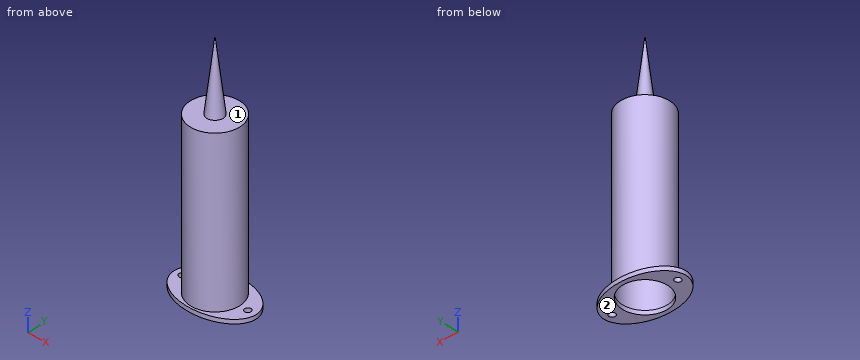
from build123d import *

# Parameters (mm, degrees)
SKETCH1_R           = 19.05
SKETCH1_R_2         = 17.4625
BOSS_EXTRUDE1_DEPTH = 123.825
SKETCH2_RX          = 31.75
SKETCH2_RY          = 20.6375
SKETCH2_R           = 17.4625
SKETCH2_R_2         = 2.413
BOSS_EXTRUDE2_DEPTH = 3.175
SKETCH3_R           = 17.4625
BOSS_EXTRUDE3_DEPTH = 4.953


with BuildPart() as part:
    # Sketch1 → Boss-Extrude1 (new body)
    with BuildSketch(Plane.XY):
        Circle(SKETCH1_R)
        Circle(SKETCH1_R_2, mode=Mode.SUBTRACT)
    extrude(amount=BOSS_EXTRUDE1_DEPTH)

    # Sketch2 → Boss-Extrude2 (add)
    with BuildSketch(Plane(origin=(0, 0, 0), x_dir=(-1, 0, 0), z_dir=(0, 0, -1))):
        with Locations((0, 0)):
            Ellipse(SKETCH2_RX, SKETCH2_RY)
        Circle(SKETCH2_R, mode=Mode.SUBTRACT)
        with Locations((25.4, 0)):
            Circle(SKETCH2_R_2, mode=Mode.SUBTRACT)
        with Locations((-25.4, 0)):
            Circle(SKETCH2_R_2, mode=Mode.SUBTRACT)
    extrude(amount=BOSS_EXTRUDE2_DEPTH)

    # Sketch3 → Boss-Extrude3 (add)
    with BuildSketch(Plane.XY.offset(123.825)):
        Circle(SKETCH3_R)
    extrude(amount=-BOSS_EXTRUDE3_DEPTH)

    # Sketch4 → Revolve1 (revolve)
    with BuildSketch(Plane(origin=(0, 0, 0), x_dir=(1, 0, 0), z_dir=(0, 1, 0))):
        Polygon((0, -123.825), (0, -177.8), (6.35, -123.825), align=None)
    revolve(axis=Axis((0, 0, 123.825), (0, 0, 1)))


solid = part.part
Model file for the job. Use its own axes, mm. Face numbers are marked on the shaded views. A direction names the side the tool comes from. Round coordinates to 2 decimals unless told otherwise and drop trailing zeros. Order: outer loops, then holes, each group sorted by start corner. A loop starts at its lowest first (then second) coordinate and runs counter-clockwise, first axis right, second up. Notation, with made-up numbers: M -38,40 L -25,40 A35 cw -25,74 Z; hole C 87.25,59 d2. An arc over 180 degrees is marked long. Write each question's results on one line, items separated by ' | '. Start each with the question number.
(1) Saw through at B-B, the plane z = 159.5. Give the cut face in (x, y).
(2) Probe probe 1 along Y at (x, z) = (0, 65.5); probe 2 along Z at (x, y) = (-3, -16.5) (3 decimals); probe 3 along Z at (x, y) = (-19, -12) (3 decimals). List the from-to ranges inside material, lowest first. Write a range as from..to.
(3) Drop flat-ended pins along their axis: pin 1 (10.5 mm diameter, centred on x = -5, y = 4.5, fed in from -Z); pin 2 (5 mm diameter, centred on y = -10.5, z = 79.5, fed in from -X); pin 3 (4.5 mm diameter, centred on x = -25.4, y = 0, fed in from +Z); pin 4 (1 mm diameter, centred on y = -6, z = 31.5, fed in from -X). Give the stop position or say it passes through.
(4) Which spindle directions (+Z, -Z, +X, -X, +Y, -Y) get a long thin tool onto all of the face, cutting with end or side? Do the marked faces 1 and 2. Say none if no direction does.
Established:
1) outline: C 0,0 d4.31
2) probe 1: y = -19.05..-17.46, 17.46..19.05 | probe 2: z = 118.872..123.825 | probe 3: z = -3.175..0
3) pin 1: stops at z = 118.87 | pin 2: stops at x = -17.29 | pin 3: passes through | pin 4: stops at x = -18.24
4) face 1: +Z | face 2: -Z, +X, -X, +Y, -Y
